For this review, take the finished solid that the model builds, in its own axes (mm). A direction names the side the tool comes from. Give positions to 0.01 mm unless a question says otherwise; leave off trailing zeros. Order: outer loops, then holes, each group sorted by start corner. A loop starts at its lowest first (then second) coordinate and runs counter-clockwise, first axis right, second up. Notation, with made-up numbers: (59.25, 36) -> (116.25, 36) arc R22 cw to (116.25, 48) -> close; hole circle Ø8 at (30, -36.75). An arc over 180 degrees is marked (long way). One line per item, written item: value. Start each with the question number.
from build123d import *

# Parameters (mm, degrees)
SKETCH_1_R      = 2.5
SKETCH_1_R_2    = 8
EXTRUDE_1_DEPTH = 10
SKETCH_2_R      = 14
SKETCH_2_R_2    = 8
EXTRUDE_2_DEPTH = 30


with BuildPart() as part:
    # 草图1 → 凸台-拉伸1 (new body)
    with BuildSketch(Plane.XY):
        with BuildLine():
            Line((20, 13.266499161), (20, -13.266499161))
            ThreePointArc((20, -13.266499161), (0, -24), (-20, -13.266499161))
            Line((-20, -13.266499161), (-20, 13.266499161))
            ThreePointArc((-20, 13.266499161), (0, 24), (20, 13.266499161))
        make_face()
        with Locations((0, 19)):
            Circle(SKETCH_1_R, mode=Mode.SUBTRACT)
        with Locations((13.435028843, 13.435028843)):
            Circle(SKETCH_1_R, mode=Mode.SUBTRACT)
        with Locations((-13.435028843, 13.435028843)):
            Circle(SKETCH_1_R, mode=Mode.SUBTRACT)
        with Locations(Location((0, -19, 0), (0, 0, 180))):
            Circle(SKETCH_1_R, mode=Mode.SUBTRACT)
        with Locations(Location((-13.435028843, -13.435028843, 0), (0, 0, 180))):
            Circle(SKETCH_1_R, mode=Mode.SUBTRACT)
        with Locations(Location((13.435028843, -13.435028843, 0), (0, 0, 180))):
            Circle(SKETCH_1_R, mode=Mode.SUBTRACT)
        Circle(SKETCH_1_R_2, mode=Mode.SUBTRACT)
    extrude(amount=EXTRUDE_1_DEPTH)

    # 草图2 → 凸台-拉伸2 (add)
    with BuildSketch(Plane.XY.offset(10)):
        Circle(SKETCH_2_R)
        Circle(SKETCH_2_R_2, mode=Mode.SUBTRACT)
    extrude(amount=EXTRUDE_2_DEPTH)


solid = part.part
Q1. For line 1 along X through (y, z) = (18.5, 6); line 2 along Y through (x, z) = (-7, 23.5); line 3 along Y through (x, z) = (15, 4) (3 decimals), list the stretches that pass through material, from the lowest coordinate up.
Q2. Take a section at B-B (x = 0). State the section outline as (y, z) points.
Q3. For pin 1 Ø4 at (x, y) = (13.44, -13.44) entering from -Z; pin 2 Ø1 at (y, z) = (5, 35) entering from +X; pin 3 Ø8 at (x, y) = (13.44, 13.44) entering from +Z; pin 4 Ø1.5 at (x, z) = (5, 10) entering from -Y, all flat-tipped, find the tip position at first contact; note any pin that passes through.
Q4. For faces 1 (the cylindrical face through (12.932, -5.362, 24.79)), 2 (the cylindrical face through (15.82, 14.19, 4.93)), list the 3-axis set-ups (+Z, -Z, +X, -X, +Y, -Y) from which the entire face can be reached by the end or side of a thin tool; tool diameter is ignored.
Q5. Take a section at C-C (z = 23.5). State the section outline as (x, y) points.
Q6. Take a section at A-A (y = 0). State the section outline as (x, z) points, and give its area (3 significant figures).
Q7. Mouldability with a two-part tool opening along Y and no side actions: class faces 3 (the cylindrical face through (11, -14, 5)), 4 (the flat face through (20, 0, 5)), 5 (the cylindrical face through (0, 24, 5)) as pulls with the +Y half, pulls with the -Y half, needs draft (parallel to the pull), parting line crosses it, or undercut.
Q8. Take a section at D-D (x = -10). State the section outline as (y, z) points.
Answers below:
1. line 1: x = -15.29 to -2.45, 2.45 to 15.29
1. line 2: y = -12.12 to -3.87, 3.87 to 12.12
1. line 3: y = -18.735 to -15.385, -11.485 to 11.485, 15.385 to 18.735
2. outline: (-24, 0) -> (-21.5, 0) -> (-21.5, 10) -> (-24, 10) -> close; (-16.5, 0) -> (-8, 0) -> (-8, 40) -> (-14, 40) -> (-14, 10) -> (-16.5, 10) -> close; (8, 0) -> (16.5, 0) -> (16.5, 10) -> (14, 10) -> (14, 40) -> (8, 40) -> close; (21.5, 0) -> (24, 0) -> (24, 10) -> (21.5, 10) -> close
3. pin 1: passes through
3. pin 2: stops at x = 13.26
3. pin 3: stops at z = 10
3. pin 4: stops at y = -23.62
4. face 1: +Z
4. face 2: +Z, -Z
5. outline: circle Ø28 at (0, 0); hole circle Ø16 at (0, 0)
6. outline: (-20, 0) -> (-8, 0) -> (-8, 40) -> (-14, 40) -> (-14, 10) -> (-20, 10) -> close; (8, 0) -> (20, 0) -> (20, 10) -> (14, 10) -> (14, 40) -> (8, 40) -> close
6. area: 600 mm²
7. face 3: undercut
7. face 4: needs draft
7. face 5: pulls with the +Y half
8. outline: (-21.82, 0) -> (21.82, 0) -> (21.82, 10) -> (9.8, 10) -> (9.8, 40) -> (-9.8, 40) -> (-9.8, 10) -> (-21.82, 10) -> close
